Model file for the job. Use its own axes, mm. Coordinates: 2 decimals unless noted, no trailing zeros. Write each loop counter-clockwise with the first axis right and the second up, starting at its lowest first coordinate (ties: lowest second). Pieces come first, ordered by that corner, then holes. Notation, with made-up numbers: (11, 60) - (58, 60) arc R26 cw to (58, 92) - close; hole circle Ø6 at (67.5, 14). An arc over 180 degrees is marked (long way). Put each result on its own line as item: value. Start each with the question number.
1. Saw through at C-C, the plane z = 0.15. Write the cut outline in (x, y), plus the area to 3 significant figures.
2. Drill centre lines: L1, parallel to X at y = 0, z = 0.35; L2, parallel to X at y = 1.25, z = 0.25; L3, parallel to Y at x = -12.5, z = 0.85. Where is each one in solid material? Low to high. Write a range as from..to.
3. Drop a flat-ended pin along its axis: P1, Ø2.5, axis at x = 53.5, y = 0, coming from the +Z side. Give the stop position or say it passes through.
4. Saw through at B-B, the plane x = -85. Write the cut outline in (y, z).
5. Saw through at D-D, the plane x = -66.5. Write the cut outline in (y, z).
6. Saw through at A-A, the plane y = 0. Write the cut outline in (x, z).
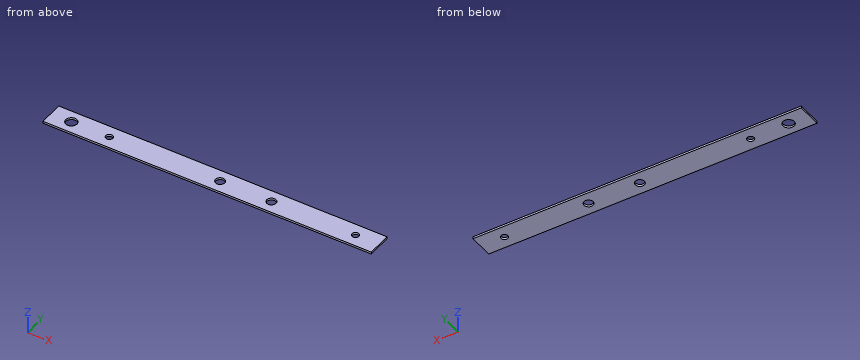
Autodesk Inventor part; units mm, degrees
ref_plane "YZ Plane" through (0, 0, 0) normal (1, 0, 0) x (0, 1, 0)
ref_plane "XZ Plane" through (0, 0, 0) normal (0, 1, 0) x (-1, 0, 0)
ref_plane "XY Plane" through (0, 0, 0) normal (0, 0, 1) x (1, 0, 0)
sketch "Sketch1" plane through (0, 0, 0) normal (0, 0, 1) x (1, 0, 0)
  line L0 (-75, -6) -> (75, -6)
  line L1 (75, -6) -> (75, 6)
  line L2 (75, 6) -> (-75, 6)
  line L3 (-75, 6) -> (-75, -6)
  line L4 (-75, -6) -> (75, 6) construction
  line L5 (75, -6) -> (-75, 6) construction
  point P0 (0, 0)
  dimension "d0" = 150
  dimension "d1" = 12
extrude "Extrusion1" add sketch "Sketch1" along normal blind 1
sketch "Sketch2" plane through (0, 0, 1) normal (0, 0, 1) x (1, 0, 0)
  line L0 (-66.5, 0) -> (-53.5, 0) construction
  line L1 (-53.5, 0) -> (53.5, 0) construction
  line L2 (53.5, 0) -> (66.5, 0) construction
  point P0 (0, 0)
  point P1 (0, 0)
  dimension "d4" = 133
  dimension "d5" = 13
  dimension "d6" = 13
hole "Hole1" at (-66.5, 0, 1) at (53.5, 0, 1) direction (0, 0, -1) diameter 3.4 depth 8 tip angle 118
sketch "Sketch4" plane through (0, 0, 1) normal (0, 0, 1) x (1, 0, 0)
  line L0 (-12.5, 0) -> (12.5, 0) construction
  point P0 (0, 0)
  point P1 (0, 0)
  dimension "d21" = 25
hole "Hole3" at (-12.5, 0, 1) at (12.5, 0, 1) direction (0, 0, -1) diameter 4.5 depth 8 tip angle 118
sketch "Sketch6" plane through (-75, -6, 0) normal (-1, 0, 0) x (0, 0, 1)
  line L0 (1, 0) -> (1, 12)
  line L1 (0, 0) -> (1, 0)
  line L2 (1, 0) -> (1, 12)
  line L3 (1, 12) -> (0, 12)
  line L4 (0, 12) -> (0, 0)
  point P0 (0, 6)
extrude "Extrusion2" add sketch "Sketch6" along normal blind 20
sketch "Sketch7" plane through (0, 0, 1) normal (0, 0, 1) x (1, 0, 0)
  line L0 (-95, -6) -> (-95, 6)
  point P0 (0, 0)
  point P1 (-85, 0)
  dimension "d39" = 10
hole "Hole5" at (-85, 0, 1) direction (0, 0, -1) diameter 5.5 depth 8 tip angle 118
sketch "Sketch8" plane through (0, 0, 1) normal (0, 0, 1) x (1, 0, 0)
  line L0 (75, -6) -> (-95, -6)
  line L1 (75, 6) -> (-95, 6)
  line L2 (75, -6) -> (65, -6)
  line L3 (65, -6) -> (65, 6)
  line L4 (65, 6) -> (75, 6)
  line L5 (75, 6) -> (75, -6)
  point P0 (0, 0)
  dimension "d47" = 10
extrude "Extrusion3" cut sketch "Sketch8" against normal blind 10
properties part number "CU6" material "Copper"
Final values:
1. outline: (-95, -6) - (65, -6) - (65, 6) - (-95, 6) - close; hole circle Ø5.5 at (-85, 0); hole circle Ø3.4 at (-66.5, 0); hole circle Ø4.5 at (-12.5, 0); hole circle Ø4.5 at (12.5, 0); hole circle Ø3.4 at (53.5, 0)
1. area: 1,850 mm²
2. L1: x = -95..-87.75, -82.25..-68.2, -64.8..-14.75, -10.25..10.25, 14.75..51.8, 55.2..65
2. L2: x = -95..-87.45, -82.55..-67.65, -65.35..-14.37, -10.63..10.63, 14.37..52.35, 54.65..65
2. L3: y = -6..-2.25, 2.25..6
3. P1: passes through
4. outline: (-6, 0) - (-2.75, 0) - (-2.75, 1) - (-6, 1) - close; (2.75, 0) - (6, 0) - (6, 1) - (2.75, 1) - close
5. outline: (-6, 0) - (-1.7, 0) - (-1.7, 1) - (-6, 1) - close; (1.7, 0) - (6, 0) - (6, 1) - (1.7, 1) - close
6. outline: (-95, 0) - (-87.75, 0) - (-87.75, 1) - (-95, 1) - close; (-82.25, 0) - (-68.2, 0) - (-68.2, 1) - (-82.25, 1) - close; (-64.8, 0) - (-14.75, 0) - (-14.75, 1) - (-64.8, 1) - close; (-10.25, 0) - (10.25, 0) - (10.25, 1) - (-10.25, 1) - close; (14.75, 0) - (51.8, 0) - (51.8, 1) - (14.75, 1) - close; (55.2, 0) - (65, 0) - (65, 1) - (55.2, 1) - close
